Job drawing, mm, ordinate dimensions from the low corner. One solid piece. Give positions to 0.01 mm unless a question says otherwise; leave off trailing zeros. Order: outer loops, then holes, each group sorted by start corner. A loop starts at its lowest first (then second) coordinate and runs counter-clockwise, first axis right, second up.
Item 1: Band-saw the part on A-A on z = 27.5. Give the cut face in (x, y).
Item 2: Wall check: L1, parallel to X at y = 5.75, z = 10; L2, parallel to Y at x = 3.75, z = 12 (1 decimal); L3, parallel to Y at x = 6.5, z = 6 (1 decimal). Give the ranges that are in metal, low to high.
Item 3: Two-plate mould, pull along X, no slides. Class the marked faces 1, 2 and 3: released by +X, released by -X, zero draft, split by the parting line, or undercut.
Item 4: Flat gauge pins, fed straight in: P1, Ø3, axis at x = 2, z = 27, coming from the -Y side (1 decimal); P2, Ø6, axis at x = 5, z = 35.5, coming from the -Y side; P3, Ø3, axis at y = 10.5, z = 30.5, coming from the +X side. Where does each tip first touch, or does it go through?
Item 5: Band-saw the part on B-B on y = 10.75. Give the cut face in (x, z).
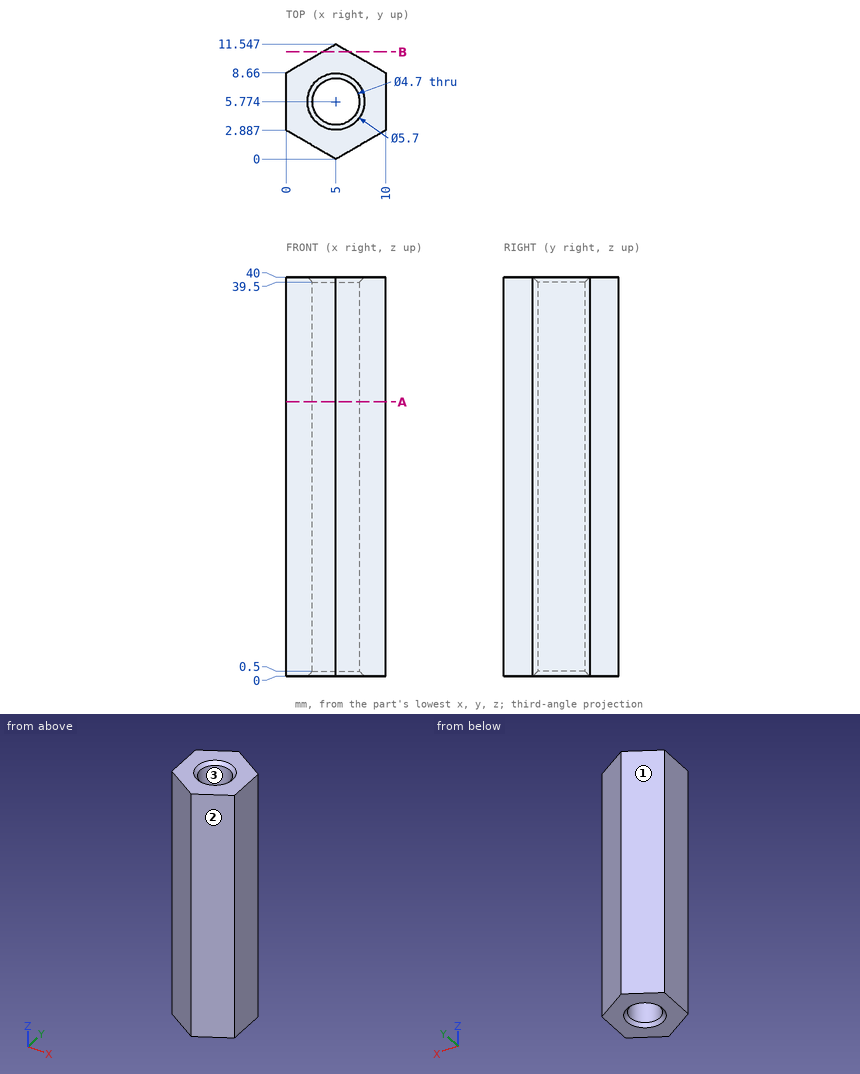
The answers:
1. outline: (0, 2.89) - (5, 0) - (10, 2.89) - (10, 8.66) - (5, 11.55) - (0, 8.66) - close; hole circle Ø4.7 at (5, 5.77)
2. L1: x = 0 to 2.65, 7.35 to 10
2. L2: y = 0.7 to 3.8, 7.8 to 10.8
2. L3: y = 0.9 to 4, 7.6 to 10.7
3. face 1: released by -X
3. face 2: released by +X
3. face 3: undercut
4. P1: stops at y = 0.9
4. P2: stops at y = 0
4. P3: stops at x = 9.41
5. outline: (3.62, 0) - (6.38, 0) - (6.38, 40) - (3.62, 40) - close
